For this review, take the finished solid that the model builds, in its own axes (mm). A direction names the side the tool comes from. Round coordinates to 2 decimals unless told otherwise and drop trailing zeros. Order: outer loops, then holes, each group sorted by start corner. A loop starts at its lowest first (then second) coordinate and runs counter-clockwise, first axis right, second up. Notation, with made-up numbers: (86.25, -23.75) -> (99.25, -23.75) arc R15 ccw to (99.25, 3.25) -> close; hole circle Ø3 at (61.25, -8.5). An arc over 180 degrees is marked (long way). Answer in a Markdown table with one row per item.
Autodesk Inventor part; units mm, degrees
ref_plane "YZ Plane" through (0, 0, 0) normal (1, 0, 0) x (0, 1, 0)
ref_plane "XZ Plane" through (0, 0, 0) normal (0, 1, 0) x (-1, 0, 0)
ref_plane "XY Plane" through (0, 0, 0) normal (0, 0, 1) x (1, 0, 0)
sketch "Sketch1" plane through (0, 0, 0) normal (0, 0, 1) x (1, 0, 0)
  line L0 (0, 0) -> (16, 0)
  line L1 (16, 0) -> (16, 1.5)
  line L2 (16, 1.5) -> (2.35, 1.5)
  line L3 (2.35, 1.5) -> (2.15, 1.5)
  line L4 (2.15, 1.5) -> (1.67, 1.5)
  line L5 (1.65, 1.515) -> (1.65, 1.515)
  line L6 (1.65, 1.515) -> (0.415, 2.75)
  line L7 (0.415, 2.75) -> (0, 2.75)
  line L8 (0, 2.75) -> (0, 0)
  line L9 (1.65, 1.515) -> (1.65, 1.52)
  arc A0 (1.65, 1.52) -> (1.67, 1.5) centre (1.67, 1.52) ccw
  dimension "d17" = 16
  dimension "d18" = 0.415
  dimension "d19" = 1.65
  dimension "d20" = 0
  dimension "d21" = 5.5
  dimension "d22" = 3
  dimension "d23" = 3
  dimension "d25" = 45
  dimension "d26" = 0.2
  dimension "d28" = 0.02
  dimension "d29" = 13.65
  dimension "d30" = 0.02
  dimension "d52" = 0.7
revolve "Revolution1" add sketch "Sketch1" angle 360 about axis through (0, 0, 0) along (1, 0, 0)
thread "Thread1"
sketch "Sketch2" plane through (0, 0, 0) normal (-1, 0, 0) x (0, 0, 1)
  circle A0 centre (0, 0) radius 1.4 construction
  circle A1 centre (0, 0) radius 0.98 construction
  line L0 (0, 0) -> (0.8487, 0.49)
  line L1 (0, 0) -> (0.98, 0) construction
  line L2 (0, 0) -> (0.8487, -0.49)
  line L3 (0, 0) -> (0.98, 0) construction
  line L4 (0.8487, 0.49) -> (1.4, 0)
  line L5 (1.4, 0) -> (0.8487, -0.49)
  dimension "d34" = 2.8
  dimension "d35" = 1.96
  dimension "d39" = 30
  dimension "d40" = 330
extrude "Extrusion1" cut sketch "Sketch2" against normal blind 0.83
pattern_circular "Circular Pattern1" count 6 over 360 about axis through (-10, 0, 0) along (1, 0, 0) of "Extrusion1"
fillet "Fillet1" radius 0.3 12 edges at (0.415, 0.49, 0.8487) (0.415, 0, 1.4) (0.415, -0.49, 0.8487) (0.415, -0.98, 0) (0.415, -1.2124, 0.7) (0.415, -1.2124, -0.7) (0.415, -0.49, -0.8487) (0.415, 0, -1.4) (0.415, 0.49, -0.8487) (0.415, 1.2124, -0.7) (0.415, 0.98, 0) (0.415, 1.2124, 0.7)
equation "\"d32\" = b"
equation "\"d34\" = A_"
equation "\"d35\" = 0.7 * A_"
equation "\"d43\" = t"
equation "\"d48\" = v"
equation "\"d17\" = l_"
equation "\"d18\" = 0.5 * t"
equation "\"d19\" = k"
equation "\"d21\" = dk"
equation "\"d22\" = d"
equation "\"d23\" = ds_"
equation "\"d25\" = 0.5 * headAngle"
equation "\"d26\" = x"
equation "\"d28\" = r"
equation "\"d29\" = b"
properties part number "Šroub se zápustnou hlavou a šestiramennou drážkou ISO 14581 - M3x16-4.8" material "Ocel, měkká"
Q1. Clearance check with a flat-ended pin moving along its axis: pin 1 Ø0.7 at (y, z) = (-0.5, 0) entering from -X. State where the tip first meets the part, or that it passes through.
Answer key:
| item | result |
|---|---|
| pin 1 | stops at x = 0.83 |
Q2. Take a section at A-A, the plane y = 0. Write out the cut boundary in (x, z) (3 decimals), then the cut area to 3 significant figures.
Answer key:
| item | result |
|---|---|
| outline | (0, -2.75) -> (0.415, -2.75) -> (1.65, -1.515) arc R0.02 cw to (1.67, -1.5) -> (16, -1.5) -> (16, 1.5) -> (1.67, 1.5) arc R0.02 cw to (1.651, 1.515) -> (0.415, 2.75) -> (0, 2.75) -> (0, 1.248) -> (0.83, 1.248) -> (0.83, -1.248) -> (0, -1.248) -> close |
| area | 48.5 mm^2 |
Q3. Take a section at B-B, the plane x = 8.25. Write out the cut boundary in (y, z).
Answer key:
| item | result |
|---|---|
| outline | circle Ø3 at (0, 0) |
Q4. To check wall thickness, follow probe 1 along Y at (x, z) = (5, 1.25); probe 2 along X at (y, z) = (1.4, 1.8); probe 3 along X at (y, z) = (-0.05, -0.05). State the ranges of each line that lie inside material, in increasing order.
Answer key:
| item | result |
|---|---|
| probe 1 | y = -0.83 to 0.83 |
| probe 2 | x = 0 to 0.88 |
| probe 3 | x = 0.83 to 16 |
Q5. Tool access review of faces 1 (the face through (16, 0, 0)), 2 (the face through (0.83, 0, 0)), 3 (the face through (8.73, -1.5, -0.07)): name each direction out of +Z, -Z, +X, -X, +Y, -Y from which nothing blocks a thin tool from reaching the whole face with its end or side.
Answer key:
| item | result |
|---|---|
| face 1 | +Z, -Z, +X, +Y, -Y |
| face 2 | -X |
| face 3 | +X |
